```python
from build123d import *

# Parameters (mm, degrees)
BOSS_EXTRUDE1_DEPTH        = 3
F_3_8_0_3750_DOWEL_HOLE1_D = 9.525


with BuildPart() as part:
    # Sketch1 → Boss-Extrude1 (new body)
    with BuildSketch(Plane.XY):
        Polygon((-50.625, 0), (-50.625, -44), (-20.625, -44), (-20.625, -49), (20.625, -49), (20.625, -44), (50.625, -44), (50.625, 0), align=None)
    extrude(amount=BOSS_EXTRUDE1_DEPTH)

    # 3/8 (0.3750) Dowel Hole1 (through all)
    with Locations(Plane.XY.offset(3)):
        with Locations((0, -22)):
            Hole(F_3_8_0_3750_DOWEL_HOLE1_D / 2)


solid = part.part
```
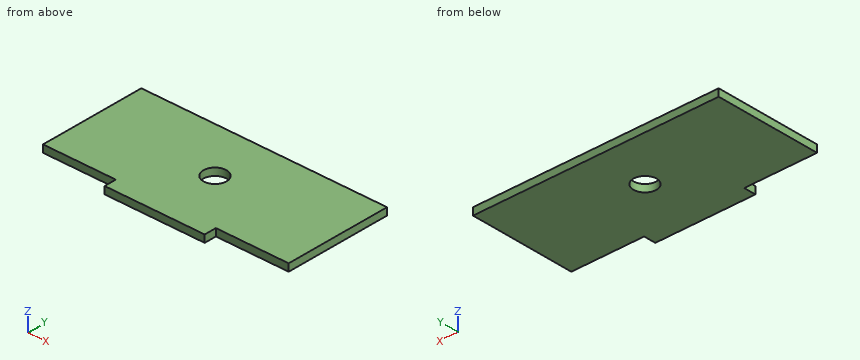
Can you work these out from the model? Positions are in its coordinate system, mm. Round coordinates to 2 decimals unless told otherwise and drop trailing zeros. Loops run counter-clockwise (first coordinate to the right, second up) from the corner with the lowest first, then second, coordinate; pieces in that order, holes last. Notation, with made-up numbers: (34, 32.5) -> (76, 32.5) arc R8 ccw to (76, 43.5) -> close; hole circle Ø7 at (-16, -12.5). An arc over 180 degrees is marked (long way). Answer in a Markdown table with one row per item.
Item 1: Suppose I cut it at C-C, the plane z = 1.25. List the corners of the cut face in (x, y) for me (1 decimal), plus the area to 3 significant figures.
Answer block:
| item | result |
|---|---|
| outline | (-50.6, -44) -> (-20.6, -44) -> (-20.6, -49) -> (20.6, -49) -> (20.6, -44) -> (50.6, -44) -> (50.6, 0) -> (-50.6, 0) -> close; hole circle Ø9.5 at (0, -22) |
| area | 4,590 mm² |
Item 2: If I drill on probe 1 along Y at (x, z) = (0, 1); probe 2 along Y at (x, z) = (2, 1.5); probe 3 along Y at (x, z) = (-44, 2.5), over which ranges is the centre line in solid material (lowest first)?
Answer block:
| item | result |
|---|---|
| probe 1 | -49 to -26.76, -17.24 to 0 |
| probe 2 | -49 to -26.32, -17.68 to 0 |
| probe 3 | -44 to 0 |
Item 3: Suppose I cut it at D-D, the plane x = -43.5. List the corners of the cut face in (y, z) for me, plus the area to 3 significant figures.
Answer block:
| item | result |
|---|---|
| outline | (-44, 0) -> (0, 0) -> (0, 3) -> (-44, 3) -> close |
| area | 132 mm² |
Item 4: Suppose I cut it at A-A, the plane x = 0. List the corners of the cut face in (y, z) for me, plus the area to 3 significant figures.
Answer block:
| item | result |
|---|---|
| outline | (-49, 0) -> (-26.76, 0) -> (-26.76, 3) -> (-49, 3) -> close; (-17.24, 0) -> (0, 0) -> (0, 3) -> (-17.24, 3) -> close |
| area | 118 mm² |
Item 5: Will these pins go through, and if not, where does the flat tip stop? P1, Ø0.9, axis at x = 36.5, z = 2, coming from the -Y side; P2, Ø1.5, axis at y = -47.5, z = 2, coming from the -X side (3 decimals).
Answer block:
| item | result |
|---|---|
| P1 | y = -44 |
| P2 | x = -20.625 |
Item 6: Suppose I cut it at B-B, the plane y = -22. List the corners of the cut face in (x, z) for me (1 decimal), plus the area to 3 significant figures.
Answer block:
| item | result |
|---|---|
| outline | (-50.6, 0) -> (-4.8, 0) -> (-4.8, 3) -> (-50.6, 3) -> close; (4.8, 0) -> (50.6, 0) -> (50.6, 3) -> (4.8, 3) -> close |
| area | 275 mm² |
